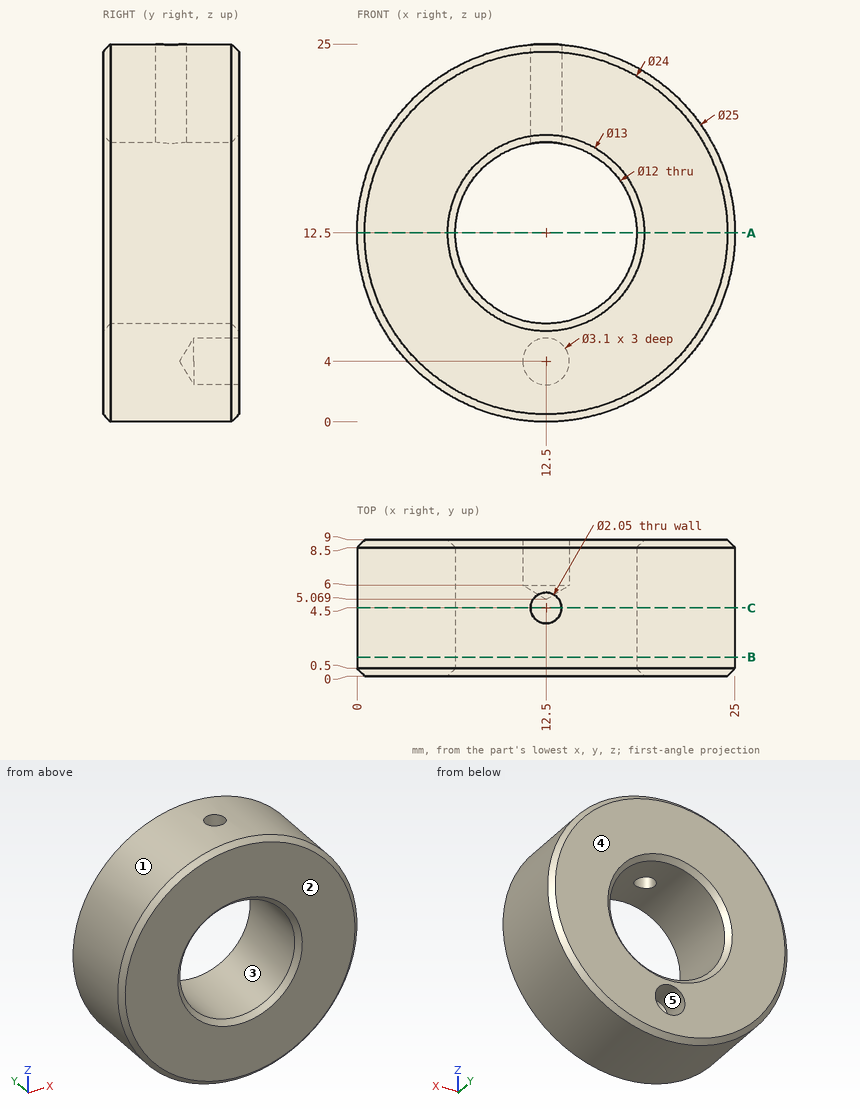
Could you check a few things on this drawing? It's one solid part, dimensions in mm from its lowest x, y, z. A direction names the side the tool comes from. Round coordinates to 2 decimals unless told otherwise and drop trailing zeros. Loops run counter-clockwise (first coordinate to the right, second up) from the corner with the lowest first, then second, coordinate; pieces in that order, holes last. Notation, with made-up numbers: M 46,30.5 L 105,30.5 A17 cw 105,59.5 Z; hole C -20,-8.75 d2. An arc over 180 degrees is marked long. Write item = value, one per line. Start each with the question number.
(1) Suppose I cut it at B-B on y = 1.25. Write out the boundary of the cut face in (x, z), plus the area to 3 significant figures.
(2) I'm going to push flat-ended pins straight in: P1, Ø9.5, axis at x = 12.5, z = 12.5, coming from the -Y side; P2, Ø1.5, axis at x = 13, z = 18, coming from the -Y side; P3, Ø4, axis at x = 5, y = 3.5, coming from the +Z side (1 decimal); P4, Ø4, axis at y = 5, z = 2.5, coming from the -X side (1 decimal). Where does each tip first touch, or does it pass through?
(3) Which directions (+Z, -Z, +X, -X, +Y, -Y) give clear straight access to the entire face, cutting with the end or side of a thin tool? Please do the marked faces 4 and 5.
(4) Suppose I cut it at C-C on y = 4.5. Write out the boundary of the cut face in (x, z) (1 decimal).
(5) If we mould it in two halves opening along Z, with no side actions, what happens to the marked faces 1, 2 and 3? For each: released by +Z, released by -Z, zero draft, split by the parting line, or undercut.
(6) I need wall thicknesses on line 1 along X through (y, z) = (6.25, 12.5); line 2 along X through (y, z) = (5.25, 21.75); line 3 along Z through (x, y) = (10, 2.5) (1 decimal). Which ranges of each line are inside material? Lowest first, please.
(7) Suppose I cut it at A-A on z = 12.5. Write out the boundary of the cut face in (x, y).
Answer block:
q1.outline = C 12.5,12.5 d25; hole C 12.5,12.5 d12
q1.area = 378 mm²
q2.P1 = through
q2.P2 = 0.23
q2.P3 = 23.7
q2.P4 = 2.9
q3.face_4 = +Z, -Z, +X, -X, +Y
q3.face_5 = +Y
q4.outline = M 11.5,18.4 L 11.5,25 A12.5 ccw long 13.5,25 L 13.5,18.4 A6 cw long Z
q5.face_1 = split by the parting line
q5.face_2 = zero draft
q5.face_3 = undercut
q6.line_1 = 0 to 6.5, 18.5 to 25
q6.line_2 = 4.09 to 11.8, 13.2 to 20.91
q6.line_3 = 0.3 to 7, 18 to 24.7
q7.outline = M 0,0.5 L 0.5,0 L 6,0 L 6.5,0.5 L 6.5,8.5 L 6,9 L 0.5,9 L 0,8.5 Z; M 18.5,0.5 L 19,0 L 24.5,0 L 25,0.5 L 25,8.5 L 24.5,9 L 19,9 L 18.5,8.5 Z
